Could you check a few things on this model? Use its own coordinates, in mm. Coordinates: 2 decimals unless noted, no trailing zeros. Loops run counter-clockwise (first coordinate to the right, second up) from the corner with the lowest first, then second, coordinate; pieces in that order, holes last. Notation, with made-up numbers: (5, 0.5) - (33, 0.5) arc R12 cw to (33, 14.5) - close; hole circle Ø6 at (32, 87). An arc over 180 degrees is marked (long way). One line per item, written item: value. Start each with the question number.
(1) If I drill on line 1 along X through (y, z) = (6.75, 261); line 2 along Z through (x, y) = (-143, 6.25), over which ranges is the centre line in solid material (lowest first)? Write a range as from..to.
(2) If we section it at B-B on y = 0: Write out the boundary of the cut face in (x, z), then the cut area to 3 significant figures.
(3) I'm going to push flat-ended pins straight in: P1, Ø1, axis at y = 1.5, z = 106.5, coming from the +X side; P2, Ø15, axis at x = -94.5, z = 311, coming from the +Y side (3 decimals); P3, Ø21, axis at x = 111.5, z = 137.5, coming from the +Y side (3 decimals). Where does each tip first touch, or does it pass through?
(4) If we section it at A-A on z = 177.5: Write out the boundary of the cut face in (x, y) (1 decimal), then the cut area to 3 significant figures.
```python
from build123d import *

# Parameters (mm, degrees)
F0_W     = 366.7125
F0_H     = 438.15
F1_DEPTH = 9.525
F2_W     = 366.7125
F2_H     = 19.05
F3_DEPTH = 6.35
F4_W     = 19.05
F4_H     = 738.1875
F4_H_2   = 138.1125
F5_DEPTH = 12.7


with BuildPart() as f1:
    # F0 (on Front) → F1 (new body, symmetric)
    with BuildSketch(Plane.XZ):
        with Locations((-64.5477453259, 219.075)):
            Rectangle(F0_W, F0_H)
        with Locations((-64.5477453259, -219.075)):
            Rectangle(F0_W, F0_H)
    extrude(amount=F1_DEPTH, both=True)

    # F2 (on face) → F3 (cut)
    with BuildSketch(Plane(origin=(0, 9.525, 0), x_dir=(-1, 0, 0), z_dir=(0, 1, 0))):
        with Locations((64.5477453259, 309.5625)):
            Rectangle(F2_W, F2_H)
    extrude(amount=-F3_DEPTH, mode=Mode.SUBTRACT)

    # F4 (on face) → F5 (cut)
    with BuildSketch(Plane(origin=(0, 9.525, 0), x_dir=(-1, 0, 0), z_dir=(0, 1, 0))):
        with Locations((-109.2835046741, -69.05625)):
            Rectangle(F4_W, F4_H)
        with Locations((-109.2835046741, 369.09375)):
            Rectangle(F4_W, F4_H_2)
        with Locations((238.3789953259, 369.09375)):
            Rectangle(F4_W, F4_H_2)
        with Locations((238.3789953259, -69.05625)):
            Rectangle(F4_W, F4_H)
    extrude(amount=-F5_DEPTH, mode=Mode.SUBTRACT)


solid = f1.part
```
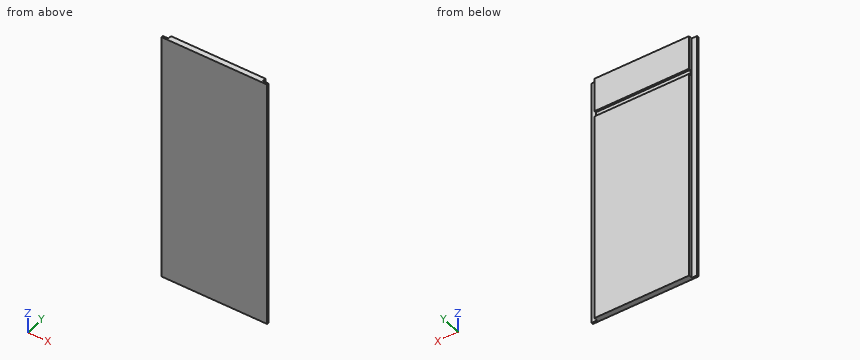
Values:
1. line 1: x = -228.85..99.76
1. line 2: z = -438.15..300.04, 319.09..438.15
2. outline: (-228.85, -438.15) - (99.76, -438.15) - (99.76, 438.15) - (-228.85, 438.15) - close
2. area: 288,000 mm2
3. P1: stops at x = 99.76
3. P2: stops at y = 3.175
3. P3: stops at y = -3.175
4. outline: (-247.9, -9.5) - (118.8, -9.5) - (118.8, -3.2) - (99.8, -3.2) - (99.8, 9.5) - (-228.9, 9.5) - (-228.9, -3.2) - (-247.9, -3.2) - close
4. area: 6,500 mm2
